Print and shaded views of the part. All mm, measured from the part's lowest x, y and z. A direction names the side the tool comes from. Round coordinates to 2 decimals unless told otherwise and drop trailing zeros. Order: outer loops, then holes, each group sorted by start corner. A loop starts at its lowest first (then second) coordinate and runs counter-clockwise, first axis right, second up. Notation, with made-up numbers: (-19.5, 18) - (-6.5, 18) arc R21 ccw to (-6.5, 53) - close; hole circle Ø6 at (55, -3.75). An arc over 180 degrees is marked (long way). Write item = value, one per line. Start each with the question number.
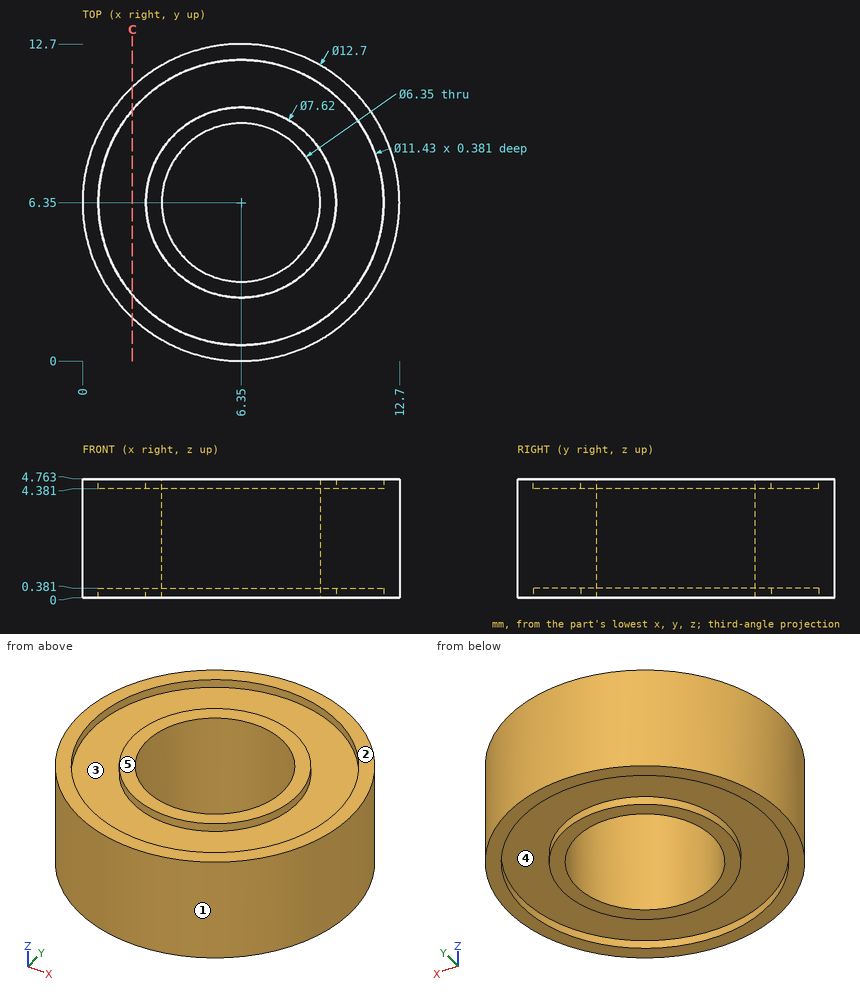
Item 1: Probe L1, parallel to Y at x = 6.35, z = 0.2 (1 decimal); L2, parallel to Y at x = 6, z = 4.5 (1 decimal); L3, parallel to Y at x = 6.35, z = 1.85 (1 decimal). List the from-to ranges inside material, lowest first.
Item 2: Drop a flat-ended pin along its axis: pin 1 (2 mm diameter, centred on x = 9, z = 2, fed in from +Y). Give the stop position or say it passes through.
Item 3: Which spindle directions (+Z, -Z, +X, -X, +Y, -Y) get a long thin tool onto all of the face, cutting with end or side? Do the marked faces 4 and 5. Say none if no direction does.
Item 4: Saw through at C-C, the plane x = 2. Give the cut face in (y, z), then the cut area to 3 significant figures.
Item 5: Mould opens along Y. For the marked faces 1, 2 and 3 say: +Y half, -Y half, draft (parallel to the pull), parting line (faces both ways), or undercut.
Check sheet entries:
q1.L1 = 0 to 0.6, 2.5 to 3.2, 9.5 to 10.2, 12.1 to 12.7
q1.L2 = 0 to 0.6, 2.6 to 3.2, 9.5 to 10.1, 12.1 to 12.7
q1.L3 = 0 to 3.2, 9.5 to 12.7
q2.pin_1 = 12.48
q3.face_4 = -Z
q3.face_5 = +Z, +X, -X, +Y, -Y
q4.outline = (1.72, 0) - (2.64, 0) - (2.64, 0.38) - (10.06, 0.38) - (10.06, 0) - (10.98, 0) - (10.98, 4.76) - (10.06, 4.76) - (10.06, 4.38) - (2.64, 4.38) - (2.64, 4.76) - (1.72, 4.76) - close
q4.area = 38.4 mm2
q5.face_1 = parting line
q5.face_2 = draft
q5.face_3 = undercut
